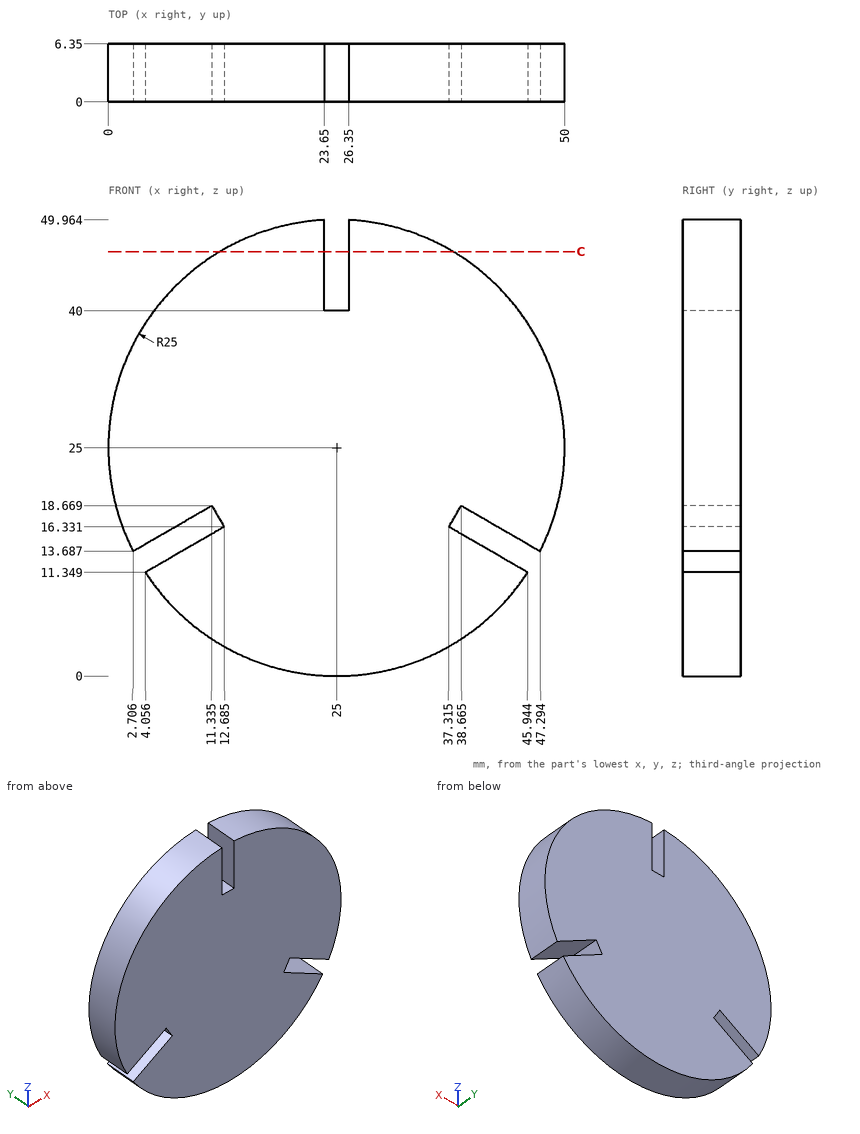
Input: dimensioned drawing with shaded views. Units: mm. Origin: part minimum x, y, z. Give positions to 0.01 mm unless a question says otherwise; leave off trailing zeros. Write each loop counter-clockwise with the first axis right and the second up, starting at its lowest first coordinate (ties: lowest second). Pieces come first, ordered by that corner, then holes.
Q1. First-contact query: P1, Ø12, axis at x = 43, z = 14, coming from the +Y side; P2, Ø1.9, axis at y = 4, z = 45.5, coming from the -X side; P3, Ø3, axis at y = 3.5, z = 46, coming from the +X side (1 decimal); P4, Ø1, axis at y = 4.5, z = 22, coming from the -X side (1 decimal). Flat tips, straight axial feed; report the tip coordinate or a pass-through.
Q2. Section C-C, the plane z = 46.5. Output: boundary loops of the cut face in (x, y), plus the area to 3 significant figures.
Q3. Material intervals for probe 1 along Z at (x, y) = (40, 1.75); probe 2 along X at (y, z) = (4, 16) (1 decimal); probe 3 along Z at (x, y) = (9, 1.5) (1 decimal), sorted ascending.
Filled in:
1. P1: stops at y = 6.35
1. P2: stops at x = 9.42
1. P3: stops at x = 40.6
1. P4: stops at x = 0.1
2. outline: (12.24, 0) - (23.65, 0) - (23.65, 6.35) - (12.24, 6.35) - close; (26.35, 0) - (37.76, 0) - (37.76, 6.35) - (26.35, 6.35) - close
2. area: 145 mm2
3. probe 1: z = 5 to 14.78, 17.9 to 45
3. probe 2: x = 1.7 to 6.7, 12.1 to 37.9, 43.3 to 48.3
3. probe 3: z = 5.8 to 14.2, 17.3 to 44.2
